```python
from build123d import *

# Parameters (mm, degrees)
SKETCH1_W           = 40
SKETCH1_H           = 25
BOSS_EXTRUDE1_DEPTH = 300
FILLET1_RADIUS      = 12.5
FILLET1_LENGTH      = 300
FILLET2_RADIUS      = 12.5
FILLET2_LENGTH      = 300
CHAMFER1_SIZE       = 5
SKETCH3_R           = 3
CUT_EXTRUDE2_DEPTH  = 304.685692781


with BuildPart() as part:
    # Sketch1 → Boss-Extrude1 (new body)
    with BuildSketch(Plane(origin=(0, 0, 0), x_dir=(1, 0, 0), z_dir=(0, 1, 0))):
        with Locations((20, 12.5)):
            Rectangle(SKETCH1_W, SKETCH1_H)
    extrude(amount=BOSS_EXTRUDE1_DEPTH)

    # Fillet1: full round fillet: the end face becomes a half cylinder, R = half its width
    fillet1_face = Plane((40, 150, -12.5), x_dir=(0, 1, 0), z_dir=(1, 0, 0))  # on the end face: x along it, z out of the body
    fillet1_slab = fillet1_face.offset(-FILLET1_RADIUS / 2) * Box(FILLET1_LENGTH, 2 * FILLET1_RADIUS, FILLET1_RADIUS, mode=Mode.PRIVATE)  # the body's end, R deep
    fillet1_round = Plane((27.5, 150, -12.5), x_dir=(1, 0, 0), z_dir=(0, 1, 0)) * Cylinder(FILLET1_RADIUS, FILLET1_LENGTH, mode=Mode.PRIVATE)  # its axis R under the face
    add(fillet1_slab - fillet1_round, mode=Mode.SUBTRACT)

    # Fillet2: full round fillet: the end face becomes a half cylinder, R = half its width
    fillet2_face = Plane((0, 150, -12.5), x_dir=(0, 1, 0), z_dir=(-1, 0, 0))  # on the end face: x along it, z out of the body
    fillet2_slab = fillet2_face.offset(-FILLET2_RADIUS / 2) * Box(FILLET2_LENGTH, 2 * FILLET2_RADIUS, FILLET2_RADIUS, mode=Mode.PRIVATE)  # the body's end, R deep
    fillet2_round = Plane((12.5, 150, -12.5), x_dir=(-1, 0, 0), z_dir=(0, 1, 0)) * Cylinder(FILLET2_RADIUS, FILLET2_LENGTH, mode=Mode.PRIVATE)  # its axis R under the face
    add(fillet2_slab - fillet2_round, mode=Mode.SUBTRACT)

    # Chamfer1
    chamfer1_edges = [part.edges().sort_by_distance(p)[0] for p in [
        (20, 300, -25),
        (40, 300, -12.5),
        (20, 300, 0),
        (0, 300, -12.5),
    ]]
    chamfer(chamfer1_edges, length=CHAMFER1_SIZE)

    # Sketch3 → Cut-Extrude2 (cut, through all)
    with BuildSketch(Plane.XY):
        with Locations((20, 268)):
            Circle(SKETCH3_R)
    extrude(amount=-CUT_EXTRUDE2_DEPTH, mode=Mode.SUBTRACT)


solid = part.part
```
Read the model definition and answer for the solid it produces. Units are mm, in the model's axes. Coordinates: 2 decimals unless noted, no trailing zeros. Loops run counter-clockwise (first coordinate to the right, second up) from the corner with the lowest first, then second, coordinate; pieces in that order, holes last. Notation, with made-up numbers: (20.5, -16) -> (41.5, -16) arc R22 cw to (41.5, 18) -> close; hole circle Ø2 at (89, 78). An arc over 180 degrees is marked (long way). Return JSON: item names as keys, results as strings.
Item 1: Find the intervals of material crossed by probe 1 along Y at (x, z) = (20, -17); probe 2 along X at (y, z) = (268, -11.5); probe 3 along Y at (x, z) = (21, -3.75), in increasing order.
Answers:
{"probe 1": "y = 0 to 265, 271 to 300", "probe 2": "x = 0.04 to 17, 23 to 39.96", "probe 3": "y = 0 to 265.17, 270.83 to 298.75"}
Item 2: Find section C-C (y = 212.5). Determine the outline of the cut face in (x, z), plus the area to 3 significant figures.
Answers:
{"outline": "(12.5, -25) -> (27.5, -25) arc R12.5 ccw to (27.5, 0) -> (12.5, 0) arc R12.5 ccw to start", "area": "866 mm2"}
Item 3: Find section A-A (x = 20). Determine the outline of the cut face in (y, z), plus the area to 4 significant figures.
Answers:
{"outline": "(0, -25) -> (265, -25) -> (265, 0) -> (0, 0) -> close; (271, -25) -> (295, -25) -> (300, -20) -> (300, -5) -> (295, 0) -> (271, 0) -> close", "area": "7,325 mm2"}
Item 4: Find section B-B (y = 268). Determine the outline of the cut face in (x, z).
Answers:
{"outline": "(12.5, -25) -> (17, -25) -> (17, 0) -> (12.5, 0) arc R12.5 ccw to start; (23, -25) -> (27.5, -25) arc R12.5 ccw to (27.5, 0) -> (23, 0) -> close"}
Item 5: Flat-ended cylindrical pins translate along their axes: P1, Ø1, axis at y = 86, z = -19, coming from the +X side; P2, Ø5, axis at y = 253, z = -6, coming from the -X side; P3, Ø10, axis at y = 236, z = -5, coming from the +X side. Find the tip coordinate at first contact, or state that the pin passes through.
Answers:
{"P1": "stops at x = 38.47", "P2": "stops at x = 0.66", "P3": "stops at x = 39.75"}
Item 6: For a pull along X with two mould halves and no side action, classify faces 1 (the conical face through (4.2, 299.2, -12.3)), 2 (the flat face through (20, 145, -25)), 3 (the conical face through (35.8, 299.2, -12.7)), 4 (the cylindrical face through (20, 271, -12)) as +X half, -X half, draft (parallel to the pull), parting line (faces both ways), or undercut.
Answers:
{"face 1": "-X half", "face 2": "draft", "face 3": "+X half", "face 4": "undercut"}
